Source: CAD feature listing. Evaluate the final solid. Frame: model axes, mm. A direction names the side the tool comes from. Round coordinates to 2 decimals unless told otherwise and drop trailing zeros. Write each loop counter-clockwise with the first axis right and the second up, starting at its lowest first coordinate (ties: lowest second). Pieces come first, ordered by that corner, then holes. Notation, with made-up numbers: M -12,46.25 L 24,46.25 A12 ccw 24,51.25 Z; hole C 83,85.25 d1. An arc over 180 degrees is marked long. Put each result on its own line as item: value. Start each with the question number.
```python
from build123d import *

# Parameters (mm, degrees)
RUNROUTE_R           = 17.9
RUNEXTRUDE_DEPTH     = 25.6
OUTLETROUTE_R        = 17.9
OUTLETEXTRUDE_DEPTH  = 25.6
TEESHELL_START       = -25.6
TEESHELL_OUTLINE_R   = 16
TEESHELL_DEPTH       = 51.2
TEESHELL_START_2     = -1e-07
TEESHELL_2_OUTLINE_R = 16
TEESHELL_2_DEPTH     = 25.6000001
TEECHAMFER_SIZE      = 0.633333333


with BuildPart() as part:
    # RunRoute → RunExtrude (new body)
    with BuildSketch(Plane(origin=(0, 0, 0), x_dir=(0, 0, -1), z_dir=(1, 0, 0))):
        Circle(RUNROUTE_R)
    runextrude = extrude(amount=RUNEXTRUDE_DEPTH)

    # RunExtrudeMirror: RunExtrude across plane
    add(runextrude.mirror(Plane(origin=(0, 0, 0), x_dir=(0, 0, 1), z_dir=(1, 0, 0))))

    # OutletRoute → OutletExtrude (add)
    with BuildSketch(Plane(origin=(0, 0, 0), x_dir=(1, 0, 0), z_dir=(0, 1, 0))):
        with Locations(Location((0, 0, 0), (0, 0, 270))):
            Circle(OUTLETROUTE_R)
    extrude(amount=OUTLETEXTRUDE_DEPTH)

    # TeeShell: read off the stored shape, not the designer's step
    # TeeShell outline → TeeShell (cut)
    with BuildSketch(Plane.YZ.offset(TEESHELL_START)):
        Circle(TEESHELL_OUTLINE_R)
    extrude(amount=TEESHELL_DEPTH, mode=Mode.SUBTRACT)

    # TeeShell 2 outline → TeeShell 2 (cut)
    with BuildSketch(Plane(origin=(0, 0, 0), x_dir=(1, 0, 0), z_dir=(0, 1, 0)).offset(TEESHELL_START_2)):
        Circle(TEESHELL_2_OUTLINE_R)
    extrude(amount=TEESHELL_2_DEPTH, mode=Mode.SUBTRACT)

    # TeeChamfer
    # the kernel refuses this chamfer: 0.633333333 mm, written as the material it takes off along each edge
    with BuildSketch(Plane(origin=(25.6, 0, 0), x_dir=(0, 0, -1), z_dir=(0, -1, 0))) as teechamfer_piece_1:
        Polygon((17.9, -TEECHAMFER_SIZE), (17.9 - TEECHAMFER_SIZE, 0), (17.9, 0), align=None)
    revolve(axis=Axis((25.6, 0, 0), (1, 0, 0)), mode=Mode.SUBTRACT)
    with BuildSketch(Plane(origin=(-25.6, 0, 0), x_dir=(0, 0, -1), z_dir=(0, -1, 0))) as teechamfer_piece_2:
        Polygon((17.9, TEECHAMFER_SIZE), (17.9 - TEECHAMFER_SIZE, 0), (17.9, 0), align=None)
    revolve(axis=Axis((-25.6, 0, 0), (1, 0, 0)), mode=Mode.SUBTRACT)
    with BuildSketch(Plane(origin=(0, 25.6, 0), x_dir=(0, 0, 1), z_dir=(-1, 0, 0))) as teechamfer_piece_3:
        Polygon((17.9, -TEECHAMFER_SIZE), (17.9 - TEECHAMFER_SIZE, 0), (17.9, 0), align=None)
    revolve(axis=Axis((0, 25.6, 0), (0, 1, 0)), mode=Mode.SUBTRACT)


solid = part.part
```
(1) Contact query for flat-ended pins moving along their axis: P1, Ø10, axis at x = 15, y = 10.5, coming from the +Z side; P2, Ø3, axis at y = 12, z = 5, coming from the -X side; P3, Ø3, axis at x = 11, y = 3.5, coming from the -Z side; P4, Ø1.5, axis at x = -20.5, y = 16.5, coming from the -Z side. Output: stop coordinate, or through.
(2) Ray query, line 1 along Z through (x, y) = (0, 18.25); line 2 along Y through (x, z) = (-21.5, -2). Return the intervals inside material, ascending.
(3) Section query C-C (x = -21.5). Return loops of the section in (y, z), and give its area (3 significant figures).
(4) Pull-direction query (X, two-part tool) for faces 1 (the cylindrical face through (15.26, 18.31, -4.81)), 2 (the flat face through (-25.6, -11.43, -11.43)), 3 (the cylindrical face through (0.787, 17.857, -17.883)), 4 (the flat face through (-11.43, 25.6, 11.43)); classes: +X half, -X half, draft (parallel to the pull), parting line (faces both ways), or undercut.
(5) Access query for faces 5 (the cylindrical face through (-0.358, -15.985, 0.703)), 6 (the cylindrical face through (0.35, -17.474, 3.88)). Directions: +Z, -Z, +X, -X, +Y, -Y. A direction counts if a zero-diameter tool reaches every point of the face in a straight line with its end or side. Return the directions, or none.
(6) Section query A-A (z = 0). Return loops of the section in (x, y), and give its area (3 significant figures).
(7) Section query B-B (x = 0). Return loops of the section in (y, z).
(8) Section query D-D (z = -8.5). Count the separate pieces of the cut face and the enclosed holes in it, and give its area (3 significant figures).
Entries:
1. P1: z = 17.03
1. P2: through
1. P3: z = -17.79
1. P4: z = -8.51
2. line 1: -17.9 to -16, 16 to 17.9
2. line 2: -17.79 to -15.87, 15.87 to 17.79
3. outline: C 0,0 d35.8; hole C 0,0 d32
3. area: 202 mm2
4. face 1: undercut
4. face 2: -X half
4. face 3: parting line
4. face 4: draft
5. face 5: +X, -X
5. face 6: none
6. outline: M -25.6,-17.27 L -24.97,-17.9 L 24.97,-17.9 L 25.6,-17.27 L 25.6,-16 L -25.6,-16 Z; M -25.6,16 L -16,16 L -16,25.6 L -17.27,25.6 L -17.9,24.97 L -17.9,17.9 L -24.97,17.9 L -25.6,17.27 Z; M 16,16 L 25.6,16 L 25.6,17.27 L 24.97,17.9 L 17.9,17.9 L 17.9,24.97 L 17.27,25.6 L 16,25.6 Z
6. area: 162 mm2
7. outline: M 0,-17.9 L 24.97,-17.9 L 25.6,-17.27 L 25.6,-16 L 0,-16 A16 cw 0,16 L 25.6,16 L 25.6,17.27 L 24.97,17.9 L 0,17.9 A17.9 ccw Z
8. separate pieces: 3
8. enclosed holes: 0
8. area: 207 mm2
